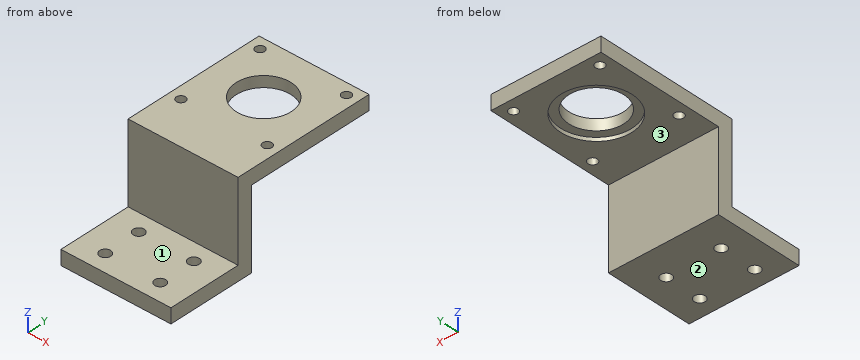
Autodesk Inventor part; units mm, degrees
ref_plane "YZ Plane" through (0, 0, 0) normal (1, 0, 0) x (0, 1, 0)
ref_plane "XZ Plane" through (0, 0, 0) normal (0, 1, 0) x (-1, 0, 0)
ref_plane "XY Plane" through (0, 0, 0) normal (0, 0, 1) x (1, 0, 0)
sketch "Szkic1" plane through (0, 0, 0) normal (0, 0, 1) x (1, 0, 0)
  line L0 (-30, -35) -> (30, -35)
  line L1 (30, -35) -> (30, 35)
  line L2 (30, 35) -> (-30, 35)
  line L3 (-30, 35) -> (-30, -35)
  line L4 (-30, -35) -> (30, 35) construction
  line L5 (30, -35) -> (-30, 35) construction
  point P0 (0, 0)
  dimension "d0" = 60
  dimension "d1" = 70
extrude "Wyciągnięcie proste1" add sketch "Szkic1" along normal blind 8
sketch "Szkic2" plane through (0, 0, 0) normal (0, 0, -1) x (-1, 0, 0)
  line L0 (30, -35) -> (-30, -35)
  line L1 (30, 35) -> (30, -35)
  line L2 (-30, 35) -> (30, 35)
  line L3 (-30, -35) -> (-30, 35)
  line L4 (23.57, 5) -> (23.57, 28.57)
  line L5 (23.57, 28.57) -> (-23.57, 28.57)
  line L6 (-23.57, 28.57) -> (-23.57, -18.57)
  line L7 (-23.57, -18.57) -> (23.57, -18.57)
  line L8 (23.57, -18.57) -> (23.57, 5)
  circle A0 centre (23.57, 28.57) radius 2.5
  circle A1 centre (-23.57, 28.57) radius 2.5
  circle A2 centre (-23.57, -18.57) radius 2.5
  circle A3 centre (23.57, -18.57) radius 2.5
  line L9 (0, 0) -> (0, 5)
  dimension "d6" = 47.14
  dimension "d7" = 47.14
  dimension "d8" = 47.14
  dimension "d9" = 5
  dimension "d10" = 5
  dimension "d11" = 5
  dimension "d12" = 5
  dimension "d15" = 5
extrude "Wyciągnięcie proste3" cut sketch "Szkic2" against normal up to next contours A0 L5 L4 | L4 L5 A0 | A3 L7 L8 | L8 L7 A3 | A1 L6 L5 | L5 L6 A1 | A2 L6 L7 | L7 L6 A2
sketch "Szkic4" plane through (0, 0, 8) normal (0, 0, 1) x (1, 0, 0)
  line L0 (-30, -35) -> (30, -35)
  line L1 (30, -35) -> (30, -43)
  line L2 (30, -43) -> (-30, -43)
  line L3 (-30, -43) -> (-30, -35)
  point P0 (0, 0)
  dimension "d18" = 8
extrude "Wyciągnięcie proste4" add sketch "Szkic4" against normal blind 43.4
sketch "Szkic5" plane through (0, 0, 8) normal (0, 0, 1) x (1, 0, 0)
  circle A0 centre (-23.57, -18.57) radius 2.5
  circle A1 centre (23.57, 28.57) radius 2.5
  circle A2 centre (-23.57, 28.57) radius 2.5
  circle A3 centre (23.57, -18.57) radius 2.5
  line L0 (30, 35) -> (30, -43)
  line L1 (30, 35) -> (-30, 35)
  line L2 (-30, 35) -> (-30, -43)
  line L3 (30, -43) -> (-30, -43)
  line L4 (23.57, -18.57) -> (-23.57, 28.57)
  line L5 (-23.57, -18.57) -> (23.57, 28.57)
  circle A4 centre (0, 5) radius 15
  point P0 (0, 0)
  dimension "d21" = 30
extrude "Wyciągnięcie proste5" cut sketch "Szkic5" against normal up to next contours A4 L4 L5 | L5 L4 A4 | L5 A4 L4 | L4 A4 L5
thread "Gwint1"
thread "Gwint2"
thread "Gwint3"
thread "Gwint4"
sketch "Szkic8" plane through (-30, -35, 0) normal (0, 1, 0) x (1, 0, 0)
  line L0 (0, 35.4) -> (60, 35.4)
  line L1 (0, 35.4) -> (0, 43.4)
  line L2 (0, 43.4) -> (60, 43.4)
  line L3 (60, 43.4) -> (60, 35.4)
  point P0 (30, 0)
  dimension "d46" = 8
extrude "Wyciągnięcie proste8" add sketch "Szkic8" against normal blind 48
sketch "Szkic9" plane through (30, -35, -43.4) normal (0, 0, -1) x (-1, 0, 0)
  line L0 (0, 0) -> (60, 0)
  line L1 (0, 0) -> (0, -48)
  line L2 (60, -48) -> (0, -48)
  line L3 (60, 0) -> (60, -48)
  line L4 (60, -8) -> (60, -48)
  line L5 (60, -48) -> (60, -38)
  line L6 (60, -38) -> (0, -38)
  line L7 (60, -38) -> (60, -18)
  line L8 (60, -18) -> (0, -18)
  line L9 (0, -8) -> (0, -48)
  line L10 (0, -48) -> (15, -48)
  line L11 (0, -48) -> (60, -48)
  line L12 (15, -48) -> (15, -18)
  line L13 (60, -48) -> (45, -48)
  line L14 (45, -48) -> (45, -18)
  circle A0 centre (45, -38) radius 3
  circle A1 centre (15, -38) radius 3
  circle A2 centre (45, -18) radius 3
  circle A3 centre (15, -18) radius 3
  point P0 (30, 35)
  dimension "d49" = 10
  dimension "d50" = 20
  dimension "d51" = 15
  dimension "d52" = 15
  dimension "d53" = 6
  dimension "d54" = 6
  dimension "d55" = 6
  dimension "d56" = 6
extrude "Wyciągnięcie proste9" cut sketch "Szkic9" against normal up to next contours A3 L8 | L8 L12 A3 | A2 L14 L8 | L8 A2 | A1 L12 L6 | L6 L12 A1 | L8 A3 L12 | A0 L14 L6 | L6 L14 A0 | L14 A2 L8 | L12 A1 L6 | L6 A1 L12 | L14 A0 L6 | L6 A0 L14
sketch "Szkic10" plane through (0, 0, 0) normal (0, 0, -1) x (-1, 0, 0)
  circle A0 centre (0, 5) radius 15
  circle A1 centre (0, 5) radius 19.5
  point P0 (0, 0)
  dimension "d59" = 39
extrude "Wyciągnięcie proste10" cut sketch "Szkic10" against normal blind 2
properties part number "Uchwyt silnika krokowego osi Y"
Here's how the part is built. I have some questions about the finished solid (model axes, mm). Face numbers are marked on the shaded views. A direction names the side the tool comes from. Round coordinates to 2 decimals unless told otherwise and drop trailing zeros. Write each loop counter-clockwise with the first axis right and the second up, starting at its lowest first coordinate (ties: lowest second). Pieces come first, ordered by that corner, then holes. Notation, with made-up numbers: (54.5, 62) -> (65.5, 62) arc R27 ccw to (65.5, 100) -> close; hole circle Ø9 at (-4.75, 31). An arc over 180 degrees is marked (long way). One line per item, written item: value.
1) Suppose I cut it at A-A on x = 23.57. List the corners of the cut face in (y, z) for me.
Filled sheet:
outline: (-83, -43.4) -> (-35, -43.4) -> (-35, 0) -> (-21.07, 0) -> (-21.07, 8) -> (-43, 8) -> (-43, -35.4) -> (-83, -35.4) -> close; (-16.07, 0) -> (26.07, 0) -> (26.07, 8) -> (-16.07, 8) -> close; (31.07, 0) -> (35, 0) -> (35, 8) -> (31.07, 8) -> close
2) Suppose I cut it at B-B on y = 5. List the corners of the cut face in (x, z) for me.
Filled sheet:
outline: (-30, 0) -> (-19.5, 0) -> (-19.5, 2) -> (-15, 2) -> (-15, 8) -> (-30, 8) -> close; (15, 2) -> (19.5, 2) -> (19.5, 0) -> (30, 0) -> (30, 8) -> (15, 8) -> close
3) For the marked faces 1, 2 and 3, which set-ups out of +Z, -Z, +X, -X, +Y, -Y let a thin tool reach every point of the face, with its end or its side?
Filled sheet:
face 1: +Z, +X, -X, -Y
face 2: -Z, +X, -X, +Y, -Y
face 3: -Z, +X, -X, +Y
4) I'm going to push flat-ended pins straight in: pin 1 Ø12 at (y, z) = (-47, -22) entering from -X; pin 2 Ø13 at (x, z) = (9.5, -25.5) entering from +Y; pin 3 Ø19.5 at (x, y) = (-9, 12.5) entering from -Z; pin 4 Ø13 at (x, z) = (6.5, -13.5) entering from -Y. Where does each tip first touch, or does it pass through?
Filled sheet:
pin 1: stops at x = -30
pin 2: stops at y = -35
pin 3: stops at z = 0
pin 4: stops at y = -43
5) Suppose I cut it at D-D on x = 0. List the corners of the cut face in (y, z) for me, plus the area to 3 significant figures.
Filled sheet:
outline: (-83, -43.4) -> (-35, -43.4) -> (-35, 0) -> (-14.5, 0) -> (-14.5, 2) -> (-10, 2) -> (-10, 8) -> (-43, 8) -> (-43, -35.4) -> (-83, -35.4) -> close; (20, 2) -> (24.5, 2) -> (24.5, 0) -> (35, 0) -> (35, 8) -> (20, 8) -> close
area: 1,030 mm2
6) If I drill on line 1 (X direction, y = -18.57, z = 5.75); line 2 (Y direction, x = -15, z = -40); line 3 (Y direction, x = -23.57, z = 5), over which ranges is the centre line in solid material (lowest first)? Write a range as [from, to].
Filled sheet:
line 1: x = [-30, -26.07], [-21.07, 21.07], [26.07, 30]
line 2: y = [-83, -76], [-70, -56], [-50, -35]
line 3: y = [-43, -21.07], [-16.07, 26.07], [31.07, 35]
7) Suppose I cut it at C-C on y = -53. List the corners of the cut face in (x, z) for me, plus the area to 3 significant figures.
Filled sheet:
outline: (-30, -43.4) -> (-18, -43.4) -> (-18, -35.4) -> (-30, -35.4) -> close; (-12, -43.4) -> (12, -43.4) -> (12, -35.4) -> (-12, -35.4) -> close; (18, -43.4) -> (30, -43.4) -> (30, -35.4) -> (18, -35.4) -> close
area: 384 mm2
